Autodesk Inventor part; units mm, degrees
ref_plane "YZ Plane" through (0, 0, 0) normal (1, 0, 0) x (0, 1, 0)
ref_plane "XZ Plane" through (0, 0, 0) normal (0, 1, 0) x (-1, 0, 0)
ref_plane "XY Plane" through (0, 0, 0) normal (0, 0, 1) x (1, 0, 0)
sketch "Sketch1" plane through (0, 0, 0) normal (0, 1, 0) x (-1, 0, 0)
  line L0 (44.45, 0) -> (-44.45, 0)
  line L1 (-44.45, 0) -> (-44.45, -188.9125)
  line L2 (-44.45, -188.9125) -> (44.45, -188.9125)
  line L3 (44.45, -188.9125) -> (44.45, 0)
  line L4 (12.7, -50.8) -> (-12.7, -50.8) construction
  line L5 (-12.7, -50.8) -> (-12.7, 0) construction
  line L6 (-12.7, 0) -> (12.7, 0) construction
  line L7 (12.7, 0) -> (12.7, -50.8) construction
  circle A0 centre (0, -152.4) radius 14.2875
  circle A1 centre (0, -184.15) radius 4.7625 construction
  point P0 (0, 0)
  point P1 (0, 0)
  dimension "d0" = 50.8
  dimension "d1" = 25.4
  dimension "d2" = 88.9
  dimension "d4" = 28.575
  dimension "d5" = 9.525
  dimension "d6" = 31.75
  dimension "d7" = 152.4
extrude "Extrusion1" add sketch "Sketch1" against normal blind 6.35
hole "Hole1" at (0, 0, -184.15) direction (0, -1, 0) diameter 5.1054 end through all
sketch "Sketch2" plane through (0, 0, 0) normal (0, 1, 0) x (1, 0, 0)
  circle A0 centre (0, 184.15) radius 2.5527 construction
  circle A1 centre (0, 152.4) radius 14.2875 construction
  line L0 (-44.45, 188.9125) -> (44.45, 188.9125) construction
  line L1 (44.45, 188.9125) -> (44.45, 0) construction
  line L2 (44.45, 0) -> (-44.45, 0) construction
  line L3 (-44.45, 0) -> (-44.45, 188.9125) construction
  line L4 (-44.45, 188.9125) -> (-44.45, 0) construction
  line L5 (-44.45, 157.1625) -> (-12.7, 188.9125)
  line L6 (44.45, 188.9125) -> (-44.45, 188.9125) construction
  line L7 (-12.7, 188.9125) -> (-44.45, 188.9125)
  line L8 (-44.45, 157.1625) -> (-44.45, 188.9125)
  line L9 (44.45, 188.9125) -> (12.7, 188.9125)
  line L10 (12.7, 188.9125) -> (44.45, 157.1625)
  line L11 (44.45, 157.1625) -> (44.45, 188.9125)
  line L12 (44.45, 0) -> (44.45, 188.9125) construction
  line L13 (-12.7, 188.9125) -> (12.7, 188.9125) construction
  line L14 (-44.45, 0) -> (-17.4625, 0)
  line L15 (-17.4625, 0) -> (-44.45, 76.2)
  line L16 (-44.45, 76.2) -> (-44.45, 0)
  line L17 (17.4625, 0) -> (44.45, 0)
  line L18 (44.45, 0) -> (44.45, 76.2)
  line L19 (44.45, 76.2) -> (17.4625, 0)
  line L20 (-44.45, 0) -> (44.45, 0) construction
  line L21 (-12.7, 0) -> (12.7, 0) construction
  line L22 (12.7, 0) -> (12.7, 50.8) construction
  line L23 (12.7, 50.8) -> (-12.7, 50.8) construction
  line L24 (-12.7, 50.8) -> (-12.7, 0) construction
  line L25 (17.4625, 0) -> (-17.4625, 0) construction
  point P0 (0, 0)
  point P1 (0, 188.9125)
  point P2 (0, 50.8)
  point P3 (0, 0)
  point P4 (0, 0)
  point P5 (0, 0)
  point P6 (0, 0)
  dimension "d18" = 25.4
  dimension "d19" = 31.75
  dimension "d20" = 31.75
  dimension "d21" = 25.4
  dimension "d22" = 50.8
  dimension "d23" = 34.925
  dimension "d24" = 76.2
extrude "Extrusion2" cut sketch "Sketch2" against normal through all
sketch "Sketch3" plane through (0, 0, 0) normal (0, 1, 0) x (1, 0, 0)
  line L0 (-17.4625, 0) -> (17.4625, 0) construction
  line L1 (0, 12.7) -> (0, 38.1) construction
  point P0 (0, 0)
  point P1 (0, 25.4)
  point P2 (0, 0)
  point P3 (0, 0)
  point P4 (0, 25.4)
  dimension "d27" = 12.7
  dimension "d28" = 25.4
hole "Hole2" at (0, 0, -12.7) at (0, 0, -25.4) at (0, 0, -38.1) direction (0, -1, 0) diameter 5.1054 end through all
equation "\"d20\" = d19"
properties part number "CL4-002" material "Aluminum 6061"
For this review, take the finished solid that the model builds, in its own axes (mm). Coordinates: 2 decimals unless noted, no trailing zeros. Order: outer loops, then holes, each group sorted by start corner. A loop starts at its lowest first (then second) coordinate and runs counter-clockwise, first axis right, second up. Notation, with made-up numbers: (89, 81) -> (140, 81) arc R30 cw to (140, 116) -> close; hole circle Ø8 at (-24, 40.25). An arc over 180 degrees is marked (long way). Answer as CSV lines item,"result".
Q1. We need section C-C (z = -25.4). State the section outline as (x, y) points.
Model answer:
outline,"(-26.46, -6.35) -> (-2.55, -6.35) -> (-2.55, 0) -> (-26.46, 0) -> close; (2.55, -6.35) -> (26.46, -6.35) -> (26.46, 0) -> (2.55, 0) -> close"
Q2. Clearance check with flat-ended pins moving along their axes: pin 1 Ø8 at (x, z) = (0, -38.1) entering from +Y; pin 2 Ø4.5 at (x, z) = (0, -184.15) entering from +Y; pin 3 Ø3 at (x, y) = (-25.5, -1.5) entering from -Z. State where each tip first meets the part, or that it passes through.
Model answer:
pin 1,"stops at y = 0"
pin 2,"passes through"
pin 3,"stops at z = -177.61"
Q3. We need section B-B (y = -3.25). Count the separate pieces of the cut face and the enclosed holes in it, plus the area to 3 significant figures.
Model answer:
separate pieces,"1"
enclosed holes,"5"
area,"13,000 mm2"
Q4. Wall thickness on line 1 along Z through (x, y) = (0, -4.5); line 2 along X through (y, z) = (-1.5, -184.15); line 3 along X through (y, z) = (-5.5, -148): over which ranges is each line inside the solid? List them lowest first. Write a range as [from, to].
Model answer:
line 1,"z = [-188.91, -186.7], [-181.6, -166.69], [-138.11, -40.65], [-35.55, -27.95], [-22.85, -15.25], [-10.15, 0]"
line 2,"x = [-17.46, -2.55], [2.55, 17.46]"
line 3,"x = [-44.45, -13.59], [13.59, 44.45]"
Q5. Draft analysis for pull direction X (two halves, no side actions). For faces 1 (the face through (1, -6.35, -93)), 2 (the face through (-0.11, -3.22, -40.65)), 3 (the face through (1.86, -3.131, -138.234)), 4 (the face through (44.45, -3, -116)), state which applies: released by +X, released by -X, zero draft, split by the parting line, or undercut.
Model answer:
face 1,"zero draft"
face 2,"undercut"
face 3,"undercut"
face 4,"released by +X"
Q6. We need section D-D (z = -45). State the section outline as (x, y) points, plus the area to 3 significant figures.
Model answer:
outline,"(-33.4, -6.35) -> (33.4, -6.35) -> (33.4, 0) -> (-33.4, 0) -> close"
area,"424 mm2"
Q7. We need section A-A (z = -152.4). State the section outline as (x, y) points.
Model answer:
outline,"(-44.45, -6.35) -> (-14.29, -6.35) -> (-14.29, 0) -> (-44.45, 0) -> close; (14.29, -6.35) -> (44.45, -6.35) -> (44.45, 0) -> (14.29, 0) -> close"
